Read the model definition and answer for the solid it produces. Units are mm, in the model's axes. A direction names the side the tool comes from. Give positions to 0.01 mm unless a question says otherwise; leave off trailing zeros. Order: outer loops, then holes, each group sorted by start corner. A loop starts at its lowest first (then second) coordinate and runs counter-clockwise, first axis right, second up. Notation, with made-up numbers: (39.25, -23) - (73.25, -23) arc R26 cw to (73.25, -4) - close; hole circle Ø3 at (-16.75, 70.25). An arc over 180 degrees is marked (long way). Use a Markdown table: item, result. Add a question column.
1. Which of the six approach directions +Z, -Z, +X, -X, +Y, -Y give full straight-line access (tool end or side, diameter ignored) to faces 1 (the cylindrical face through (-30.852, 20.923, 0.506)), 2 (the flat face through (-25, 12, 0)), 3 (the flat face through (-59, 20, -25)), 4 (the flat face through (-8, 11, 2))?
2. For a pull along X with two mould halves and no side action, classify faces 5 (the cylindrical face through (-73.58, 22.535, -26.615)), 6 (the flat face through (-13, 15.9, 2)), 7 (the flat face through (-58, 25, -11)), 8 (the flat face through (-56, 12, -18)) as released by +X, released by -X, zero draft, split by the parting line, or undercut.
3. Flat-ended cylindrical pins translate along their axes: P1, Ø1.5, axis at x = -49, y = 11, coming from the -Z side; P2, Ø12.5, axis at x = -36, y = 13, coming from the -Z side; P3, Ø3, axis at x = -33, y = 1.5, coming from the -Z side; P4, Ø3, axis at x = -71, z = -24.25, coming from the +Y side. Find the tip coordinate at first contact, or state that the pin passes through.
4. A cutting plane is placed at A-A on y = 15. Determine the outline of the cut face in (x, z).
5. A cutting plane is placed at D-D on y = 21.4. Determine the outline of the cut face in (x, z) (3 decimals).
6. Consider L1, parallel to X at y = 4.5, z = -24.25; L2, parallel to X at y = 21.45, z = -24.25; L3, parallel to Y at x = -33, z = 0.45. Determine where each line is inside the solid, lowest interval first.
7. A cutting plane is placed at C-C on y = 11.4. Determine the outline of the cut face in (x, z) (3 decimals), and give its area (3 significant figures).
8. A cutting plane is placed at B-B on x = -61. Determine the outline of the cut face in (y, z), and give its area (3 significant figures).
```python
from build123d import *

# Parameters (mm, degrees)
BOSS_EXTRUDE1_DEPTH                          = 25
SKETCH2_W                                    = 10
SKETCH2_H                                    = 9
CUT_EXTRUDE1_DEPTH                           = 87.261593424
CBORE_FOR_M3_PAN_HEAD_SCREW1_D               = 3.4
CBORE_FOR_M3_PAN_HEAD_SCREW1_CBORE_D         = 7
CBORE_FOR_M3_PAN_HEAD_SCREW1_CBORE_DEPTH     = 5
CBORE_FOR_M2_HEX_SOCKET_HEAD_CAP_SCR_2_COUNT = 2
CBORE_FOR_M2_HEX_SOCKET_HEAD_CAP_SCR_2_PITCH = 20.008001599
CBORE_FOR_M2_HEX_SOCKET_HEAD_CAP_SCR_3_COUNT = 2
CBORE_FOR_M2_HEX_SOCKET_HEAD_CAP_SCR_3_PITCH = 31.613289927


with BuildPart() as part:
    # Sketch1 → Boss-Extrude1 (new body)
    with BuildSketch(Plane(origin=(0, 0, 0), x_dir=(1, 0, 0), z_dir=(0, 1, 0))):
        Polygon((0, 0), (0, -3), (-53.75, -3), (-76, 19.25), (-76, 29.25), (-56, 29.25), (-56, 6.321067812), (-49.678932188, 0), align=None)
    extrude(amount=BOSS_EXTRUDE1_DEPTH)

    # Sketch2 → Cut-Extrude1 (cut, through all)
    with BuildSketch(Plane.XY.offset(3)):
        with Locations((-13, 11.4)):
            Rectangle(SKETCH2_W, SKETCH2_H)
    extrude(amount=-CUT_EXTRUDE1_DEPTH, mode=Mode.SUBTRACT)

    # CBORE for M3 Pan Head Screw1 (through all)
    with Locations(Plane(origin=(0, 25, 0), x_dir=(1, 0, 0), z_dir=(0, 1, 0))):
        with Locations((-71, 24.25), (-61, 24.25)):
            CounterBoreHole(CBORE_FOR_M3_PAN_HEAD_SCREW1_D / 2, CBORE_FOR_M3_PAN_HEAD_SCREW1_CBORE_D / 2, CBORE_FOR_M3_PAN_HEAD_SCREW1_CBORE_DEPTH)

    # Sketch6 → CBORE for M2 Hex Socket Head Cap Screw1 (revolve, cut)
    with BuildSketch(Plane(origin=(-33, 21.4, 0), x_dir=(0, 1, 0), z_dir=(1, 0, 0))):
        Polygon((0, 0), (0, 3), (1.2, 3), (1.2, 1), (2.2, 1), (2.2, 0.025), (2.225, 0), align=None)
    cbore_for_m2_hex_socket_head_cap_screw1 = revolve(axis=Axis((-33, 21.4, -6.35), (0, 0, 1)), mode=Mode.SUBTRACT)

    # CBORE for M2 Hex Socket Head Cap Scr 2: CBORE for M2 Hex Socket Head Cap Screw1 ×2
    with Locations(*[Vector(-0.0003998400320129169, -0.9999999200639712, 0) * (i * CBORE_FOR_M2_HEX_SOCKET_HEAD_CAP_SCR_2_PITCH) for i in range(1, CBORE_FOR_M2_HEX_SOCKET_HEAD_CAP_SCR_2_COUNT)]):
        add(cbore_for_m2_hex_socket_head_cap_screw1, mode=Mode.SUBTRACT)

    # CBORE for M2 Hex Socket Head Cap Scr 3: CBORE for M2 Hex Socket Head Cap Screw1 ×2
    with Locations(*[Vector(0.9486516610381267, -0.31632266123312, 0) * (i * CBORE_FOR_M2_HEX_SOCKET_HEAD_CAP_SCR_3_PITCH) for i in range(1, CBORE_FOR_M2_HEX_SOCKET_HEAD_CAP_SCR_3_COUNT)]):
        add(cbore_for_m2_hex_socket_head_cap_screw1, mode=Mode.SUBTRACT)


solid = part.part
```
Output values:
| question | item | result |
|---|---|---|
| 1 | face 1 | -Z |
| 1 | face 2 | -Z, +X, +Y, -Y |
| 1 | face 3 | +Y |
| 1 | face 4 | +Z, -Z |
| 2 | face 5 | undercut |
| 2 | face 6 | undercut |
| 2 | face 7 | zero draft |
| 2 | face 8 | released by +X |
| 3 | P1 | z = -0.07 |
| 3 | P2 | z = 0 |
| 3 | P3 | z = 1 |
| 3 | P4 | through |
| 4 | outline | (-76, -29.25) - (-56, -29.25) - (-56, -6.32) - (-49.68, 0) - (-18, 0) - (-18, 3) - (-53.75, 3) - (-76, -19.25) - close; (-8, 0) - (0, 0) - (0, 3) - (-8, 3) - close; hole circle Ø3.4 at (-71, -24.25); hole circle Ø3.4 at (-61, -24.25) |
| 5 | outline | (-76, -29.25) - (-56, -29.25) - (-56, -6.321) - (-49.679, 0) - (-35.225, 0) - (-35.2, 0.025) - (-35.2, 1) - (-34.2, 1) - (-34.2, 3) - (-53.75, 3) - (-76, -19.25) - close; (-31.8, 1) - (-30.8, 1) - (-30.8, 0.025) - (-30.775, 0) - (0, 0) - (0, 3) - (-31.8, 3) - close; hole circle Ø7 at (-71, -24.25); hole circle Ø7 at (-61, -24.25) |
| 6 | L1 | -76 to -72.7, -69.3 to -62.7, -59.3 to -56 |
| 6 | L2 | -76 to -74.5, -67.5 to -64.5, -57.5 to -56 |
| 6 | L3 | 3.59 to 19.2, 23.6 to 25 |
| 7 | outline | (-76, -29.25) - (-56, -29.25) - (-56, -6.321) - (-49.679, 0) - (-18, 0) - (-18, 3) - (-53.75, 3) - (-76, -19.25) - close; (-8, 0) - (-5.235, 0) - (-5.21, 0.025) - (-5.21, 1) - (-4.21, 1) - (-4.21, 3) - (-8, 3) - close; (-1.81, 1) - (-0.81, 1) - (-0.81, 0.025) - (-0.785, 0) - (0, 0) - (0, 3) - (-1.81, 3) - close; hole circle Ø3.4 at (-71, -24.25); hole circle Ø3.4 at (-61, -24.25) |
| 7 | area | 528 mm² |
| 8 | outline | (0, -29.25) - (25, -29.25) - (25, -27.75) - (20, -27.75) - (20, -25.95) - (0, -25.95) - close; (0, -22.55) - (20, -22.55) - (20, -20.75) - (25, -20.75) - (25, -4.25) - (0, -4.25) - close |
| 8 | area | 522 mm² |
